Here's the drawing with two shaded views (mm, measured from the low corner). I have some questions. Give positions to 0.01 mm unless a question says otherwise; leave off trailing zeros. Loops run counter-clockwise (first coordinate to the right, second up) from the corner with the lowest first, then second, coordinate; pieces in that order, holes last. Notation, with made-up numbers: (76, -15) - (118, -15) arc R21 ccw to (118, 14) - close; hole circle Ø6 at (39.5, -3.5). An arc over 180 degrees is marked (long way). Use a Markdown table: item, result. Add a question column.
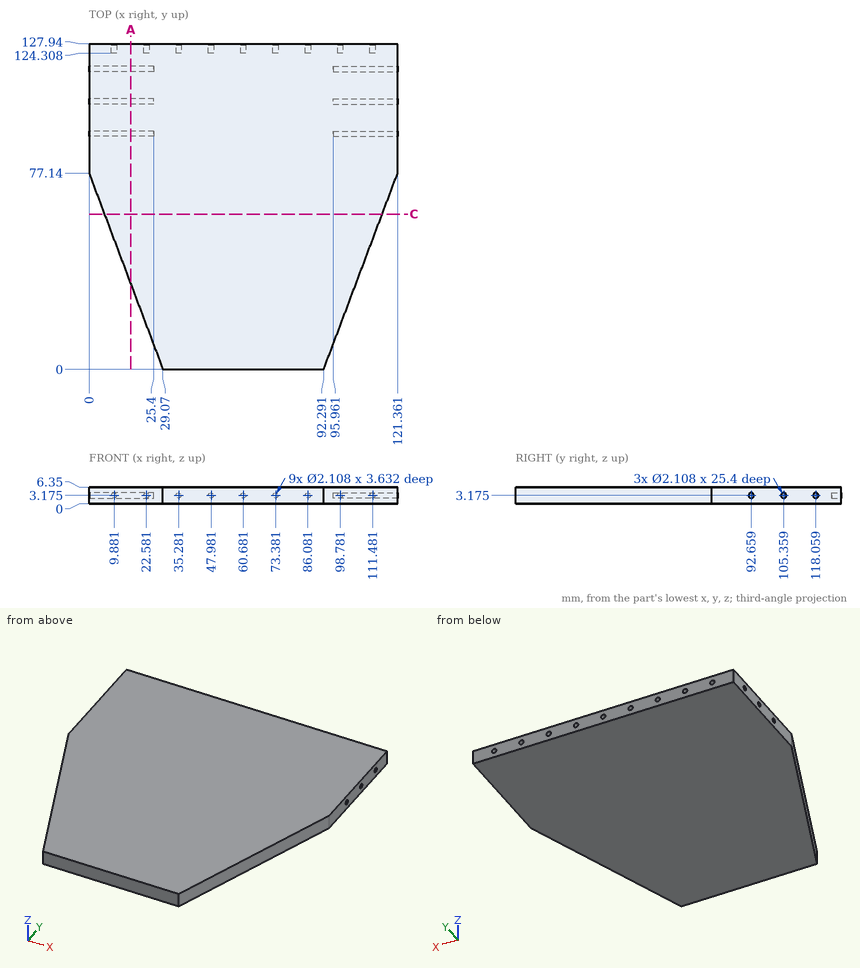
1. Will these pins go through, and if not, where does the flat tip stop? P1, Ø1.5, axis at y = 30.5, z = 4.5, coming from the -X side; P2, Ø1.1, axis at y = 105, z = 3, coming from the +X side; P3, Ø1.1, axis at x = 35, z = 3.5, coming from the +Y side.
2. Suppose I cut it at A-A (x = 16.5). State how many separate pieces and enclosed holes the cut face has, and give its area (3 significant figures).
3. Suppose I cut it at C-C (y = 61). List the corners of the cut face in (x, z) for me.
4. Please list where these lines run through material, in increasing order: line 1 along X through (y, z) = (93, 3.5); line 2 along X through (y, z) = (18.5, 1.5). Write a range as [from, to].
Results below:
| question | item | result |
|---|---|---|
| 1 | P1 | x = 17.29 |
| 1 | P2 | x = 95.96 |
| 1 | P3 | y = 124.31 |
| 2 | separate pieces | 1 |
| 2 | enclosed holes | 3 |
| 2 | area | 590 mm² |
| 3 | outline | (6.08, 0) - (115.28, 0) - (115.28, 6.35) - (6.08, 6.35) - close |
| 4 | line 1 | [25.4, 95.96] |
| 4 | line 2 | [22.1, 99.26] |
